Read the model definition and answer for the solid it produces. Units are mm, in the model's axes. Round coordinates to 2 decimals unless told otherwise and drop trailing zeros. Write each loop counter-clockwise with the first axis right and the second up, starting at its lowest first coordinate (ties: lowest second). Pieces come first, ordered by that corner, then holes. Notation, with made-up numbers: (87, 20) -> (130, 20) arc R20 ccw to (130, 52) -> close; hole circle Ø1 at (-6.5, -18). An arc over 180 degrees is marked (long way). Return JSON: item names as keys, results as strings.
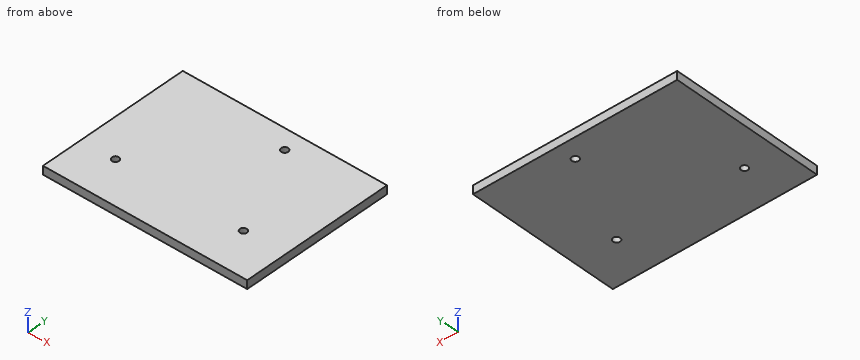
from build123d import *

# Parameters (mm, degrees)
F0_W     = 73
F0_H     = 55
F0_R     = 3.5
F0_R_2   = 1.25
F1_DEPTH = 3


# Not quite as in the source:
# - a feature names something its author has since deleted; it is built from what else it names


with BuildPart() as f1:
    # F0 (on Top) → F1 (new body)
    with BuildSketch(Plane.XY):
        with Locations((17.8632747996, -5.3606596088)):
            Rectangle(F0_W, F0_H)
        with Locations((-6.3567252004, -17.8606596088)):
            Circle(F0_R, mode=Mode.SUBTRACT)
        with BuildLine():
            ThreePointArc((39.3632747996, -14.3606596088), (41.8381485337, -15.3857858747), (42.8632747996, -17.8606596088))
            ThreePointArc((42.8632747996, -17.8606596088), (41.8381485337, -20.335533343), (39.3632747996, -21.3606596088))
            ThreePointArc((39.3632747996, -21.3606596088), (35.8632747996, -17.8606596088), (39.3632747996, -14.3606596088))
        make_face(mode=Mode.SUBTRACT)
        with Locations((24.1232747996, 15.1593403912)):
            Circle(F0_R, mode=Mode.SUBTRACT)
        with Locations((24.1232747996, 15.1593403912)):
            Circle(F0_R)
        with Locations((24.1232747996, 15.1593403912)):
            Circle(F0_R_2, mode=Mode.SUBTRACT)
        with BuildLine():
            ThreePointArc((39.3632747996, -21.3606596088), (41.8381485337, -20.335533343), (42.8632747996, -17.8606596088))
            ThreePointArc((42.8632747996, -17.8606596088), (41.8381485337, -15.3857858747), (39.3632747996, -14.3606596088))
            ThreePointArc((39.3632747996, -14.3606596088), (35.8632747996, -17.8606596088), (39.3632747996, -21.3606596088))
        make_face()
        with Locations((39.3632747996, -17.8606596088)):
            Circle(F0_R_2, mode=Mode.SUBTRACT)
        with Locations((-6.3567252004, -17.8606596088)):
            Circle(F0_R)
        with Locations((-6.3567252004, -17.8606596088)):
            Circle(F0_R_2, mode=Mode.SUBTRACT)
    extrude(amount=-F1_DEPTH)


solid = f1.part
Item 1: A flat-ended cylindrical pin translates along its axis: pin 1 (12 mm diameter, centred on x = 11.5, y = -24, fed in from +Z). Find the tip coordinate at first contact, or state that the pin passes through.
Worked answers:
{"pin 1": "stops at z = 0"}
Item 2: Section A-A (x = 24.5) is taken. Give the vertices of the cut face in (y, z), then the cut area to 3 significant figures.
Worked answers:
{"outline": "(-32.86, -3) -> (13.97, -3) -> (13.97, 0) -> (-32.86, 0) -> close; (16.35, -3) -> (22.14, -3) -> (22.14, 0) -> (16.35, 0) -> close", "area": "158 mm2"}
Item 3: Straight lines are drawn through the part: L1, parallel to X at y = -18.5, z = -1.05; L2, parallel to Y at x = 39.5, z = -0.2; L3, parallel to X at y = -17, z = -0.85. For each, find the intervals that lie inside material, in ascending order. Write a range as [from, to].
Worked answers:
{"L1": "x = [-18.64, -7.43], [-5.28, 38.29], [40.44, 54.36]", "L2": "y = [-32.86, -19.1], [-16.62, 22.14]", "L3": "x = [-18.64, -7.26], [-5.45, 38.46], [40.27, 54.36]"}
